from build123d import *

# Parameters (mm, degrees)
SKETCH1_W                = 79.8
SKETCH1_H                = 129
BOSS_EXTRUDE1_DEPTH      = 4
FILLET1_R                = 7
SKETCH2_R                = 3.325
CUT_EXTRUDE2_DEPTH       = 3.2
BOSS_EXTRUDE3_START      = 3
BOSS_EXTRUDE3_DEPTH      = 3
SKETCH6_W                = 6.35
SKETCH6_H                = 6.35
CHAMFER1_SIZE            = 1
CHAMFER1_OF_MIRROR1_SIZE = 1


with BuildPart() as part:
    # Sketch1 → Boss-Extrude1 (new body)
    with BuildSketch(Plane.XY):
        with Locations((-91.126473502, -25.83334618)):
            Rectangle(SKETCH1_W, SKETCH1_H)
    extrude(amount=BOSS_EXTRUDE1_DEPTH)

    # Fillet1
    fillet1_edges = [part.edges().sort_by_distance(p)[0] for p in [
        (-131.026473502, 38.66665382, 2),
        (-51.226473502, 38.66665382, 2),
        (-51.226473502, -90.33334618, 2),
        (-131.026473502, -90.33334618, 2),
    ]]
    fillet(fillet1_edges, radius=FILLET1_R)

    # Sketch2 → Cut-Extrude2 (cut)
    with BuildSketch(Plane(origin=(0, 0, 0), x_dir=(-1, 0, 0), z_dir=(0, 0, -1))):
        with Locations((55.726473502, 1.91665382)):
            Circle(SKETCH2_R)
        with Locations((91.126473502, 34.16665382)):
            Circle(SKETCH2_R)
        with Locations((55.726473502, -56.58334618)):
            Circle(SKETCH2_R)
        with Locations((91.126473502, -85.83334618)):
            Circle(SKETCH2_R)
        with Locations((126.526473502, 1.91665382)):
            Circle(SKETCH2_R)
        with Locations((126.526473502, -56.58334618)):
            Circle(SKETCH2_R)
    extrude(amount=-CUT_EXTRUDE2_DEPTH, mode=Mode.SUBTRACT)

    # Sketch3 → Boss-Extrude3 (add)
    # profile 1 of 3: a face of its own
    with BuildSketch(Plane.XY.offset(4).offset(BOSS_EXTRUDE3_START)):
        with BuildLine():
            Line((-136.026473502, 31.66665382), (-136.026473502, -83.33334618))
            ThreePointArc((-136.026473502, -83.33334618), (-132.511754876, -91.818627555), (-124.026473502, -95.33334618))
            Line((-124.026473502, -95.33334618), (-58.226473502, -95.33334618))
            ThreePointArc((-58.226473502, -95.33334618), (-49.741192128, -91.818627555), (-46.226473502, -83.33334618))
            Line((-46.226473502, -83.33334618), (-46.226473502, 31.66665382))
            ThreePointArc((-46.226473502, 31.66665382), (-49.741192128, 40.151935194), (-58.226473502, 43.66665382))
            Line((-58.226473502, 43.66665382), (-124.026473502, 43.66665382))
            ThreePointArc((-124.026473502, 43.66665382), (-132.511754876, 40.151935194), (-136.026473502, 31.66665382))
        make_face()
        with BuildLine():
            Line((-124.026473502, -90.33334618), (-58.226473502, -90.33334618))
            ThreePointArc((-58.226473502, -90.33334618), (-53.276726034, -88.283093649), (-51.226473502, -83.33334618))
            Line((-51.226473502, -83.33334618), (-51.226473502, 31.66665382))
            ThreePointArc((-51.226473502, 31.66665382), (-53.276726034, 36.616401288), (-58.226473502, 38.66665382))
            Line((-58.226473502, 38.66665382), (-124.026473502, 38.66665382))
            ThreePointArc((-124.026473502, 38.66665382), (-128.976220971, 36.616401288), (-131.026473502, 31.66665382))
            Line((-131.026473502, 31.66665382), (-131.026473502, -83.33334618))
            ThreePointArc((-131.026473502, -83.33334618), (-128.976220971, -88.283093649), (-124.026473502, -90.33334618))
        make_face(mode=Mode.SUBTRACT)
    # profile 2 of 3: a face of its own
    with BuildSketch(Plane.XY.offset(4).offset(BOSS_EXTRUDE3_START)):
        with BuildLine():
            ThreePointArc((-131.026473502, -83.33334618), (-128.976220971, -88.283093649), (-124.026473502, -90.33334618))
            Line((-124.026473502, -90.33334618), (-58.226473502, -90.33334618))
            ThreePointArc((-58.226473502, -90.33334618), (-53.276726034, -88.283093649), (-51.226473502, -83.33334618))
            Line((-51.226473502, -83.33334618), (-51.226473502, 31.66665382))
            ThreePointArc((-51.226473502, 31.66665382), (-53.276726034, 36.616401288), (-58.226473502, 38.66665382))
            Line((-58.226473502, 38.66665382), (-124.026473502, 38.66665382))
            ThreePointArc((-124.026473502, 38.66665382), (-128.976220971, 36.616401288), (-131.026473502, 31.66665382))
            Line((-131.026473502, 31.66665382), (-131.026473502, -83.33334618))
        make_face()
    # profile 3 of 3: a face of its own
    with BuildSketch(Plane.XY.offset(4).offset(BOSS_EXTRUDE3_START)):
        with BuildLine():
            Line((-124.026473502, -90.33334618), (-58.226473502, -90.33334618))
            ThreePointArc((-58.226473502, -90.33334618), (-53.276726034, -88.283093649), (-51.226473502, -83.33334618))
            Line((-51.226473502, -83.33334618), (-51.226473502, 31.66665382))
            ThreePointArc((-51.226473502, 31.66665382), (-53.276726034, 36.616401288), (-58.226473502, 38.66665382))
            Line((-58.226473502, 38.66665382), (-124.026473502, 38.66665382))
            ThreePointArc((-124.026473502, 38.66665382), (-128.976220971, 36.616401288), (-131.026473502, 31.66665382))
            Line((-131.026473502, 31.66665382), (-131.026473502, -83.33334618))
            ThreePointArc((-131.026473502, -83.33334618), (-128.976220971, -88.283093649), (-124.026473502, -90.33334618))
        make_face()
    extrude(amount=-BOSS_EXTRUDE3_DEPTH)

    # Sweep1: sweep along a curve in space
    with BuildLine() as sweep1_path:
        Line((-116.126473502, -10.83334618, 7), (-116.126473502, -10.83334618, 17))
        ThreePointArc((-116.126473502, -10.83334618, 17), (-114.662007408, -10.83334618, 20.535533906), (-111.126473502, -10.83334618, 22))
        Line((-111.126473502, -10.83334618, 22), (-71.126473502, -10.83334618, 22))
        ThreePointArc((-66.126473502, -10.83334618, 17), (-67.590939596, -10.83334618, 20.535533906), (-71.126473502, -10.83334618, 22))
        Line((-66.126473502, -10.83334618, 17), (-66.126473502, -10.83334618, 7))
    # Sketch6 → Sweep1 (sweep)
    with BuildSketch(Plane.XY.offset(7)):
        with Locations((-116.126473502, -10.83334618)):
            Rectangle(SKETCH6_W, SKETCH6_H)
    sweep1 = sweep(path=sweep1_path.line)

    # Chamfer1
    chamfer1_edges = [part.edges().sort_by_distance(p)[0] for p in [
        (-119.301473502, -14.00834618, 12),
        (-119.301473502, -7.65834618, 12),
        (-116.907071438, -14.00834618, 22.780597936),
        (-116.907071438, -7.65834618, 22.780597936),
        (-91.126473502, -14.00834618, 25.175),
        (-91.126473502, -7.65834618, 25.175),
        (-65.345875566, -14.00834618, 22.780597936),
        (-65.345875566, -7.65834618, 22.780597936),
        (-62.951473502, -14.00834618, 12),
        (-62.951473502, -7.65834618, 12),
    ]]
    chamfer(chamfer1_edges, length=CHAMFER1_SIZE)

    # Mirror1: Sweep1 across plane
    add(sweep1.mirror(Plane.ZX.offset(-25.83334618)))

    # Chamfer1 of Mirror1
    chamfer1_of_mirror1_edges = [part.edges().sort_by_distance(p)[0] for p in [
        (-119.301473502, -37.65834618, 12),
        (-119.301473502, -44.00834618, 12),
        (-116.907071438, -37.65834618, 22.780597936),
        (-116.907071438, -44.00834618, 22.780597936),
        (-91.126473502, -37.65834618, 25.175),
        (-91.126473502, -44.00834618, 25.175),
        (-65.345875566, -37.65834618, 22.780597936),
        (-65.345875566, -44.00834618, 22.780597936),
        (-62.951473502, -37.65834618, 12),
        (-62.951473502, -44.00834618, 12),
    ]]
    chamfer(chamfer1_of_mirror1_edges, length=CHAMFER1_OF_MIRROR1_SIZE)


solid = part.part
Design review of the part built by this model. Coordinates are the model's own, in mm. A direction names the side the tool comes from. Coordinates: 2 decimals unless noted, no trailing zeros. Loops run counter-clockwise (first coordinate to the right, second up) from the corner with the lowest first, then second, coordinate; pieces in that order, holes last.
Item 1: Clearance check with flat-ended pins moving along their axes: pin 1 (6 mm diameter, centred on x = -126.53, y = 1.92, fed in from +Z); pin 2 (10 mm diameter, centred on y = -50, z = 15, fed in from +X); pin 3 (7 mm diameter, centred on y = -42, z = 13.5, fed in from -X); pin 4 (1.2 mm diameter, centred on y = 1, z = 2, fed in from -X). State where each tip first meets the part, or that it passes through.
Completed:
pin 1: stops at z = 7
pin 2: passes through
pin 3: stops at x = -119.3
pin 4: stops at x = -131.03
Item 2: For faces 4 (the conical face through (-116.38, -7.832, 22.139)), 5 (the flat face through (-92, 38.667, 2)), 6 (the flat face through (-91, -11, 18.825)), 7 (the flat face through (-62.951, -11, 12)), 8 (the flat face through (-126, 2, 3.2)), list the 3-axis set-ups (+Z, -Z, +X, -X, +Y, -Y) from which the entire face can be reached by the end or side of a thin tool; tool diameter is ignored.
Completed:
face 4: +Z, -X, +Y
face 5: -Z, +X, -X, +Y
face 6: +Y, -Y
face 7: +Z, +X, +Y, -Y
face 8: -Z
Item 3: Draft analysis for pull direction X (two halves, no side actions). For faces 1 (the cylindrical face through (-129.03, 36.56, 2.03)), 2 (the conical face through (-66, -43.85, 22.24)), 3 (the cylindrical face through (-53.276, -54.336, 1.578)), state which applies: pulls with the +X half, pulls with the -X half, needs draft (parallel to the pull), parting line crosses it, or undercut.
Completed:
face 1: pulls with the -X half
face 2: pulls with the +X half
face 3: undercut
Item 4: Add section D-D (x = -121). Write out the cut boundary in (y, z).
Completed:
outline: (-95.33, 4) - (-90.33, 4) - (-90.33, 0) - (38.67, 0) - (38.67, 4) - (43.67, 4) - (43.67, 7) - (-95.33, 7) - close
Item 5: Add section C-C (y = -32). Write out the cut boundary in (x, z), and give its area (3 significant figures).
Completed:
outline: (-136.03, 4) - (-131.03, 4) - (-131.03, 0) - (-51.23, 0) - (-51.23, 4) - (-46.23, 4) - (-46.23, 7) - (-136.03, 7) - close
area: 589 mm2
Item 6: Add section B-B (z = 11.5). Write out the cut boundary in (x, y), and give its area (3 significant figures).
Completed:
outline: (-119.3, -43.01) - (-118.3, -44.01) - (-112.95, -44.01) - (-112.95, -37.66) - (-118.3, -37.66) - (-119.3, -38.66) - close; (-119.3, -13.01) - (-118.3, -14.01) - (-112.95, -14.01) - (-112.95, -7.66) - (-118.3, -7.66) - (-119.3, -8.66) - close; (-69.3, -44.01) - (-63.95, -44.01) - (-62.95, -43.01) - (-62.95, -38.66) - (-63.95, -37.66) - (-69.3, -37.66) - close; (-69.3, -14.01) - (-63.95, -14.01) - (-62.95, -13.01) - (-62.95, -8.66) - (-63.95, -7.66) - (-69.3, -7.66) - close
area: 157 mm2
Item 7: Add section A-A (x = -78). Write out the cut boundary in (y, z) (3 decimals), and give its area (3 significant figures).
Completed:
outline: (-95.333, 4) - (-90.333, 4) - (-90.333, 0) - (38.667, 0) - (38.667, 4) - (43.667, 4) - (43.667, 7) - (-95.333, 7) - close; (-44.008, 18.825) - (-37.658, 18.825) - (-37.658, 24.175) - (-38.658, 25.175) - (-43.008, 25.175) - (-44.008, 24.175) - close; (-14.008, 18.825) - (-7.658, 18.825) - (-7.658, 24.175) - (-8.658, 25.175) - (-13.008, 25.175) - (-14.008, 24.175) - close
area: 1,010 mm2
Item 8: Wall thickness on L1, parallel to Y at x = -113, z = 17.5; L2, parallel to Z at x = -55.5, y = -45.5; L3, parallel to Z at x = -129.5, y = -57: over which ranges is each line inside the solid? List them lowest first.
Completed:
L1: y = -44.01 to -37.66, -14.01 to -7.66
L2: z = 0 to 7
L3: z = 3.2 to 7
